Here's how the part is built. I have some questions about the finished solid (model axes, mm). A direction names the side the tool comes from. Round coordinates to 2 decimals unless told otherwise and drop trailing zeros. Order: outer loops, then holes, each group sorted by start corner. A loop starts at its lowest first (then second) coordinate and runs counter-clockwise, first axis right, second up. Notation, with made-up numbers: (-16, 5.25) - (42, 5.25) arc R21 cw to (42, 24.25) - close; hole circle Ø4 at (-32, 7). An arc over 180 degrees is marked (long way). One line per item, written item: value.
from build123d import *

# Parameters (mm, degrees)
SKETCH1_W                = 15
SKETCH1_H                = 10
BOSS_EXTRUDE1_DEPTH      = 40
BOSS_EXTRUDE2_DEPTH      = 15
BOSS_EXTRUDE2_DEPTH_BACK = 11
SKETCH3_W                = 18.791763322
SKETCH3_H                = 11.646727992
SKETCH4_W                = 12.791763322
SKETCH4_H                = 8
CUT_EXTRUDE1_DEPTH       = 43.707480201
SKETCH5_R                = 3
CUT_EXTRUDE2_DEPTH       = 44.810756502
CUT_EXTRUDE3_DEPTH       = 49.282441533
CUT_EXTRUDE3_DEPTH_BACK  = 49.282441533
SKETCH6_OUTSIDE_W        = 32.648
SKETCH6_OUTSIDE_H        = 25.502
FILLET1_R                = 10
FILLET2_R                = 1
SKETCH7_R                = 3
CUT_EXTRUDE4_DEPTH       = 45.576248719


with BuildPart() as part:
    # Sketch1 → Boss-Extrude1 (new body)
    with BuildSketch(Plane.XY):
        Rectangle(SKETCH1_W, SKETCH1_H)
    extrude(amount=BOSS_EXTRUDE1_DEPTH)

    # Sketch3 → Boss-Extrude2 (add, two sides: drawn at the far end of the back side and taken through both)
    with BuildSketch(Plane(origin=(0, 0, 0), x_dir=(-1, 0, 0), z_dir=(0, 0, -1)).offset(-BOSS_EXTRUDE2_DEPTH_BACK)):
        Rectangle(SKETCH3_W, SKETCH3_H)
    extrude(amount=BOSS_EXTRUDE2_DEPTH + BOSS_EXTRUDE2_DEPTH_BACK)

    # Sketch4 → Cut-Extrude1 (cut, through all)
    with BuildSketch(Plane(origin=(0, 5.823363996, 0), x_dir=(1, 0, 0), z_dir=(0, 1, 0))):
        with Locations((0, 11)):
            Rectangle(SKETCH4_W, SKETCH4_H)
    extrude(amount=-CUT_EXTRUDE1_DEPTH, mode=Mode.SUBTRACT)

    # Sketch5 → Cut-Extrude2 (cut, through all)
    with BuildSketch(Plane.ZY.offset(7.5)):
        with Locations(Location((35, 0, 0), (0, 0, 270))):
            Circle(SKETCH5_R)
    extrude(amount=-CUT_EXTRUDE2_DEPTH, mode=Mode.SUBTRACT)

    # Sketch6 outside → Cut-Extrude3 (cut, two sides: drawn at the far end of the back side and taken through both)
    with BuildSketch(Plane(origin=(0, 0, -7), x_dir=(-1, 0, 0), z_dir=(0, 0, -1)).offset(-CUT_EXTRUDE3_DEPTH_BACK)):
        Rectangle(SKETCH6_OUTSIDE_W, SKETCH6_OUTSIDE_H)
        with BuildLine():
            Line((-7.395881661, 5.823363996), (7.395881661, 5.823363996))
            ThreePointArc((7.395881661, 5.823363996), (8.810095223, 5.237577558), (9.395881661, 3.823363996))
            Line((9.395881661, 3.823363996), (9.395881661, -3.823363996))
            ThreePointArc((9.395881661, -3.823363996), (8.810095223, -5.237577558), (7.395881661, -5.823363996))
            Line((7.395881661, -5.823363996), (-7.395881661, -5.823363996))
            ThreePointArc((-7.395881661, -5.823363996), (-8.810095223, -5.237577558), (-9.395881661, -3.823363996))
            Line((-9.395881661, -3.823363996), (-9.395881661, 3.823363996))
            ThreePointArc((-9.395881661, 3.823363996), (-8.810095223, 5.237577558), (-7.395881661, 5.823363996))
        make_face(mode=Mode.SUBTRACT)
    extrude(amount=CUT_EXTRUDE3_DEPTH + CUT_EXTRUDE3_DEPTH_BACK, mode=Mode.SUBTRACT)

    # Fillet1
    # the kernel refuses this fillet: 10 mm, written as the material it takes off along each edge
    with BuildSketch(Plane(origin=(-7.5, 5, 11), x_dir=(1, 0, 0), z_dir=(0, 0, 1))) as fillet1_piece_1:
        with BuildLine():
            CenterArc((FILLET1_R, -FILLET1_R), FILLET1_R, 90, 90)
            Line((0, -FILLET1_R), (0, 0))
            Line((0, 0), (FILLET1_R, 0))
        make_face()
    extrude(amount=54, mode=Mode.SUBTRACT)
    with BuildSketch(Plane(origin=(7.5, 5, 11), x_dir=(-1, 0, 0), z_dir=(0, 0, 1))) as fillet1_piece_2:
        with BuildLine():
            CenterArc((FILLET1_R, FILLET1_R), FILLET1_R, 180, 90)
            Line((0, FILLET1_R), (0, 0))
            Line((0, 0), (FILLET1_R, 0))
        make_face()
    extrude(amount=54, mode=Mode.SUBTRACT)

    # Fillet2
    # the kernel refuses this fillet: 1 mm, written as the material it takes off along each edge
    with BuildSketch(Plane(origin=(-7.395881661, 3.823363996, 11), x_dir=(0, 1, 0), z_dir=(1, 0, 0))) as fillet2_piece_1:
        with BuildLine():
            CenterArc((2 - FILLET2_R, -FILLET2_R), FILLET2_R, 0, 90)
            Line((2, -FILLET2_R), (2, 0))
            Line((2, 0), (2 - FILLET2_R, 0))
        make_face()
    revolve(axis=Axis((-7.395881661, 3.823363996, 11), (0, 0, 1)), revolution_arc=90, mode=Mode.SUBTRACT)
    with BuildSketch(Plane(origin=(-9.395881661, 3.823363996, 11), x_dir=(1, 0, 0), z_dir=(0, -1, 0)), Plane(origin=(9.395881661, -3.823363996, 11), x_dir=(-1, 0, 0), z_dir=(0, 1, 0))) as fillet2_piece_2:
        with BuildLine():
            CenterArc((FILLET2_R, -FILLET2_R), FILLET2_R, 90, 90)
            Line((0, -FILLET2_R), (0, 0))
            Line((0, 0), (FILLET2_R, 0))
        make_face()
    extrude(amount=7.646727992, mode=Mode.SUBTRACT)
    with BuildSketch(Plane(origin=(-7.395881661, -3.823363996, 11), x_dir=(-1, 0, 0), z_dir=(0, 1, 0))) as fillet2_piece_3_section:
        with BuildLine():
            CenterArc((2 - FILLET2_R, -FILLET2_R), FILLET2_R, 0, 90)
            Line((2, -FILLET2_R), (2, 0))
            Line((2, 0), (2 - FILLET2_R, 0))
        make_face()
    fillet2_piece_3 = revolve(axis=Axis((-7.395881661, -3.823363996, 11), (0, 0, 1)), revolution_arc=90, mode=Mode.PRIVATE)
    fillet2_piece_3 = fillet2_piece_3 - Plane(origin=(2.5, -5, 10.778934244), x_dir=(1, 0, 0), z_dir=(0, 0, -1)) * Cylinder(10, 8, mode=Mode.PRIVATE)
    fillet2_piece_3 = split(fillet2_piece_3, bisect_by=Plane(origin=(-8.996433691, -5, 10.778934244), z_dir=(0, 1, 0)), keep=Keep.TOP, mode=Mode.PRIVATE)
    add(fillet2_piece_3, mode=Mode.SUBTRACT)
    with BuildSketch(Plane(origin=(-7.395881661, -3.823363996, 11), x_dir=(-1, 0, 0), z_dir=(0, 1, 0))) as fillet2_piece_4_section:
        with BuildLine():
            CenterArc((2 - FILLET2_R, -FILLET2_R), FILLET2_R, 0, 90)
            Line((2, -FILLET2_R), (2, 0))
            Line((2, 0), (2 - FILLET2_R, 0))
        make_face()
    fillet2_piece_4 = revolve(axis=Axis((-7.395881661, -3.823363996, 11), (0, 0, 1)), revolution_arc=90, mode=Mode.PRIVATE)
    fillet2_piece_4 = fillet2_piece_4 - Plane(origin=(2.5, -5, 10.736771206), x_dir=(1, 0, 0), z_dir=(0, 0, -1)) * Cylinder(10, 8, mode=Mode.PRIVATE)
    fillet2_piece_4 = split(fillet2_piece_4, bisect_by=Plane(origin=(-8.184472941, -5, 10.736771206), z_dir=(0, -1, 0)), keep=Keep.TOP, mode=Mode.PRIVATE)
    add(fillet2_piece_4, mode=Mode.SUBTRACT)
    with BuildSketch(Plane(origin=(-7.395881661, -3.823363996, 11), x_dir=(-1, 0, 0), z_dir=(0, 1, 0))) as fillet2_piece_5_section:
        with BuildLine():
            CenterArc((2 - FILLET2_R, -FILLET2_R), FILLET2_R, 0, 90)
            Line((2, -FILLET2_R), (2, 0))
            Line((2, 0), (2 - FILLET2_R, 0))
        make_face()
    fillet2_piece_5 = revolve(axis=Axis((-7.395881661, -3.823363996, 11), (0, 0, 1)), revolution_arc=90, mode=Mode.PRIVATE)
    fillet2_piece_5 = fillet2_piece_5 & Plane(origin=(2.5, -5, 10.786120947), x_dir=(1, 0, 0), z_dir=(0, 0, -1)) * Cylinder(10, 8, mode=Mode.PRIVATE)
    fillet2_piece_5 = split(fillet2_piece_5, bisect_by=Plane(origin=(-7.438386145, -5, 10.786120947), z_dir=(0, -1, 0)), keep=Keep.TOP, mode=Mode.PRIVATE)
    add(fillet2_piece_5, mode=Mode.SUBTRACT)
    with BuildSketch(Plane(origin=(7.395881661, -3.823363996, 11), x_dir=(0, -1, 0), z_dir=(-1, 0, 0))) as fillet2_piece_6_section:
        with BuildLine():
            CenterArc((2 - FILLET2_R, -FILLET2_R), FILLET2_R, 0, 90)
            Line((2, -FILLET2_R), (2, 0))
            Line((2, 0), (2 - FILLET2_R, 0))
        make_face()
    fillet2_piece_6 = revolve(axis=Axis((7.395881661, -3.823363996, 11), (0, 0, 1)), revolution_arc=90, mode=Mode.PRIVATE)
    fillet2_piece_6 = fillet2_piece_6 & Plane(origin=(-2.5, -5, 10.786120921), x_dir=(-1, 0, 0), z_dir=(0, 0, -1)) * Cylinder(10, 8, mode=Mode.PRIVATE)
    fillet2_piece_6 = split(fillet2_piece_6, bisect_by=Plane(origin=(7.438386148, -5, 10.786120921), z_dir=(0, -1, 0)), keep=Keep.TOP, mode=Mode.PRIVATE)
    add(fillet2_piece_6, mode=Mode.SUBTRACT)
    with BuildSketch(Plane(origin=(7.395881661, -3.823363996, 11), x_dir=(0, -1, 0), z_dir=(-1, 0, 0))) as fillet2_piece_7_section:
        with BuildLine():
            CenterArc((2 - FILLET2_R, -FILLET2_R), FILLET2_R, 0, 90)
            Line((2, -FILLET2_R), (2, 0))
            Line((2, 0), (2 - FILLET2_R, 0))
        make_face()
    fillet2_piece_7 = revolve(axis=Axis((7.395881661, -3.823363996, 11), (0, 0, 1)), revolution_arc=90, mode=Mode.PRIVATE)
    fillet2_piece_7 = fillet2_piece_7 - Plane(origin=(-2.5, -5, 10.778934427), x_dir=(-1, 0, 0), z_dir=(0, 0, -1)) * Cylinder(10, 8, mode=Mode.PRIVATE)
    fillet2_piece_7 = split(fillet2_piece_7, bisect_by=Plane(origin=(8.996433978, -5, 10.778934427), z_dir=(0, 1, 0)), keep=Keep.TOP, mode=Mode.PRIVATE)
    add(fillet2_piece_7, mode=Mode.SUBTRACT)
    with BuildSketch(Plane(origin=(7.395881661, -3.823363996, 11), x_dir=(0, -1, 0), z_dir=(-1, 0, 0))) as fillet2_piece_8_section:
        with BuildLine():
            CenterArc((2 - FILLET2_R, -FILLET2_R), FILLET2_R, 0, 90)
            Line((2, -FILLET2_R), (2, 0))
            Line((2, 0), (2 - FILLET2_R, 0))
        make_face()
    fillet2_piece_8 = revolve(axis=Axis((7.395881661, -3.823363996, 11), (0, 0, 1)), revolution_arc=90, mode=Mode.PRIVATE)
    fillet2_piece_8 = fillet2_piece_8 - Plane(origin=(-2.5, -5, 10.736771126), x_dir=(-1, 0, 0), z_dir=(0, 0, -1)) * Cylinder(10, 8, mode=Mode.PRIVATE)
    fillet2_piece_8 = split(fillet2_piece_8, bisect_by=Plane(origin=(8.184472929, -5, 10.736771126), z_dir=(0, -1, 0)), keep=Keep.TOP, mode=Mode.PRIVATE)
    add(fillet2_piece_8, mode=Mode.SUBTRACT)
    with BuildSketch(Plane(origin=(7.395881661, 3.823363996, 11), x_dir=(1, 0, 0), z_dir=(0, -1, 0))) as fillet2_piece_9:
        with BuildLine():
            CenterArc((2 - FILLET2_R, -FILLET2_R), FILLET2_R, 0, 90)
            Line((2, -FILLET2_R), (2, 0))
            Line((2, 0), (2 - FILLET2_R, 0))
        make_face()
    revolve(axis=Axis((7.395881661, 3.823363996, 11), (0, 0, 1)), revolution_arc=90, mode=Mode.SUBTRACT)
    with BuildSketch(Plane(origin=(7.395881661, 5.823363996, 11), x_dir=(0, -1, 0), z_dir=(-1, 0, 0))) as fillet2_piece_10:
        with BuildLine():
            CenterArc((FILLET2_R, -FILLET2_R), FILLET2_R, 90, 90)
            Line((0, -FILLET2_R), (0, 0))
            Line((0, 0), (FILLET2_R, 0))
        make_face()
    extrude(amount=14.791763321, mode=Mode.SUBTRACT)
    with BuildSketch(Plane(origin=(-7.395881661, -5.823363996, 11), x_dir=(0, 1, 0), z_dir=(1, 0, 0))) as fillet2_piece_11_section:
        with BuildLine():
            CenterArc((FILLET2_R, -FILLET2_R), FILLET2_R, 90, 90)
            Line((0, -FILLET2_R), (0, 0))
            Line((0, 0), (FILLET2_R, 0))
        make_face()
    fillet2_piece_11 = extrude(amount=14.791763321, mode=Mode.PRIVATE)
    fillet2_piece_11 = split(fillet2_piece_11, bisect_by=Plane(origin=(0, -5, 10.769455145), z_dir=(0, -1, 0)), keep=Keep.TOP, mode=Mode.PRIVATE)
    add(fillet2_piece_11, mode=Mode.SUBTRACT)

    # Sketch7 → Cut-Extrude4 (cut, through all)
    with BuildSketch(Plane(origin=(9.395881661, 0, 0), x_dir=(0, 0, -1), z_dir=(1, 0, 0))):
        with Locations((11.076683863, 0)):
            Circle(SKETCH7_R)
    extrude(amount=-CUT_EXTRUDE4_DEPTH, mode=Mode.SUBTRACT)


solid = part.part
Q1. We'd pull the mould along Y, two halves only. Please class faces 6 (the cylindrical face through (-8.794, 5.253, -2.325)), 7 (the flat face through (9.396, 0, 0)), 8 (the cylindrical face through (-7.875, -1.149, -13.848)): released by +Y, released by -Y, zero draft, split by the parting line, or undercut.
Results list:
face 6: released by +Y
face 7: zero draft
face 8: undercut
Q2. Will these pins go through, and if not, where does the flat tip stop? pin 1 (6 mm diameter, centred on x = 1, y = -1, fed in from -Z); pin 2 (3 mm diameter, centred on y = 1.5, z = 17.5, fed in from -X); pin 3 (7.5 mm diameter, centred on x = 1, z = 18.5, fed in from -Y).
Results list:
pin 1: z = -7
pin 2: x = -6.16
pin 3: y = -5
Q3. If we section it at A-A, the plane y = -2.5: Please give me the cut outline in (x, z) (3 decimals).
Results list:
outline: (-9.396, -15) - (-6.396, -15) - (-6.396, -12.735) - (-9.396, -12.735) - close; (-9.396, -9.418) - (-6.396, -9.418) - (-6.396, -7) - (6.396, -7) - (6.396, -9.418) - (9.396, -9.418) - (9.396, 10) arc R1 ccw to (8.396, 11) - (7.182, 11) - (7.182, 33.342) - (-7.182, 33.342) - (-7.182, 11) - (-8.396, 11) arc R1 ccw to (-9.396, 10) - close; (-7.182, 36.658) - (7.182, 36.658) - (7.182, 40) - (-7.182, 40) - close; (6.396, -15) - (9.396, -15) - (9.396, -12.735) - (6.396, -12.735) - close
Q4. If we section it at B-B, the plane z = 35: Please give me the cut outline in (x, y), then the cut area to 3 significant figures.
Results list:
outline: (-7.5, -5) - (7.5, -5) arc R10 ccw to (7.3, -3) - (-7.3, -3) arc R10 ccw to start; (-3.5, 3) - (3.5, 3) arc R10 ccw to (0, 4.68) arc R10 ccw to start
area: 36.6 mm²
Q5. If we section it at C-C, the plane x = 3.5: Please give me the cut outline in (y, z), then the cut area to 3 significant figures.
Results list:
outline: (-5.82, -7) - (5.82, -7) - (5.82, 10) arc R1 ccw to (4.82, 11) - (3, 11) - (3, 40) - (-5, 40) - (-5, 10.98) arc R1 ccw to (-5.82, 10) - close; hole circle Ø6 at (0, 35)
area: 413 mm²
Q6. Which directions (+Z, -Z, +X, -X, +Y, -Y) give clear straight access to the entire face, cutting with the end or side of a thin tool? Please do faces 1 (the flat face through (0, -5, 25)), 2 (the flat face through (0, 0, -7)), 3 (the flat face through (2, 4.4, 11)), 4 (the cylindrical face through (-5.349, 1.196, 25.289)), 5 (the flat face through (-8, 0, -15)).
Results list:
face 1: +Z, +X, -X, -Y
face 2: -Z, +Y, -Y
face 3: +Z, +Y
face 4: +Z, -X, +Y
face 5: -Z, +X, -X, +Y, -Y
Q7. If I drill on line 1 along Y through (x, z) = (-7.5, -0.5); line 2 along Z through (x, y) = (-4.25, 0); line 3 along Z through (x, y) = (-5.5, 2), over which ranges is the centre line in solid material (lowest first)?
Results list:
line 1: -5.82 to 5.82
line 2: -7 to 32, 38 to 40
line 3: -7 to 11
Q8. If we section it at D-D, the plane z = -6: Please give me the cut outline in (x, y), then the cut area to 3 significant figures.
Results list:
outline: (-9.4, -3.82) arc R2 ccw to (-7.4, -5.82) - (7.4, -5.82) arc R2 ccw to (9.4, -3.82) - (9.4, 3.82) arc R2 ccw to (7.4, 5.82) - (-7.4, 5.82) arc R2 ccw to (-9.4, 3.82) - close
area: 215 mm²
